Check sheet for the modelled part. Datum: model origin and axes. Units: mm. A direction names the side the tool comes from. Give positions to 0.01 mm unless a question says otherwise; leave off trailing zeros. Order: outer loops, then holes, each group sorted by start corner. A loop starts at its lowest first (then second) coordinate and runs counter-clockwise, first axis right, second up.
```python
from build123d import *

# Parameters (mm, degrees)
SKETCH1_W               = 139.5
SKETCH1_H               = 152.4
BOSS_EXTRUDE1_DEPTH     = 6.35
SKETCH2_W               = 139.5
SKETCH2_H               = 152.4
CUT_EXTRUDE1_DEPTH      = 3.375
SKETCH4_R               = 3.175000001
SKETCH4_R_2             = 3.175
BOSS_EXTRUDE3_DEPTH     = 12.7
SKETCH5_R               = 7.874
CUT_EXTRUDE2_DEPTH      = 16.675
SKETCH6_R               = 2.286
CUT_EXTRUDE3_DEPTH      = 3.975
SKETCH7_R               = 1.27
SKETCH7_W               = 31.75
SKETCH7_H               = 12.7
CUT_EXTRUDE4_DEPTH      = 1
CUT_EXTRUDE4_DEPTH_BACK = 16.675


with BuildPart() as part:
    # Sketch1 → Boss-Extrude1 (new body)
    with BuildSketch(Plane(origin=(0, 0, 0), x_dir=(1, 0, 0), z_dir=(0, 1, 0))):
        with Locations((69.75, 76.2)):
            Rectangle(SKETCH1_W, SKETCH1_H)
    extrude(amount=BOSS_EXTRUDE1_DEPTH)

    # Sketch2 → Cut-Extrude1 (cut)
    with BuildSketch(Plane(origin=(0, 6.35, 0), x_dir=(1, 0, 0), z_dir=(0, 1, 0))):
        with Locations((69.75, 76.2)):
            Rectangle(SKETCH2_W, SKETCH2_H)
    extrude(amount=-CUT_EXTRUDE1_DEPTH, mode=Mode.SUBTRACT)

    # Sketch4 → Boss-Extrude3 (add)
    with BuildSketch(Plane(origin=(0, 0, -152.4), x_dir=(-1, 0, 0), z_dir=(0, 0, -1))):
        with BuildLine():
            Line((-130.61, 9.325), (-130.61, 2.975))
            Line((-130.61, 2.975), (-117.91, 2.975))
            Line((-117.91, 2.975), (-117.91, 9.325))
            ThreePointArc((-117.91, 9.325), (-124.26, 15.675), (-130.61, 9.325))
        make_face()
        with Locations((-124.26, 9.325)):
            Circle(SKETCH4_R, mode=Mode.SUBTRACT)
        with BuildLine():
            Line((-21.59, 9.325), (-21.59, 2.975))
            Line((-21.59, 2.975), (-8.89, 2.975))
            Line((-8.89, 2.975), (-8.89, 9.325))
            ThreePointArc((-8.89, 9.325), (-15.24, 15.675), (-21.59, 9.325))
        make_face()
        with Locations((-15.24, 9.325)):
            Circle(SKETCH4_R_2, mode=Mode.SUBTRACT)
    extrude(amount=-BOSS_EXTRUDE3_DEPTH)

    # Sketch5 → Cut-Extrude2 (cut, through all)
    with BuildSketch(Plane.XZ):
        with Locations((69.75, -114.3)):
            Circle(SKETCH5_R)
    extrude(amount=-CUT_EXTRUDE2_DEPTH, mode=Mode.SUBTRACT)

    # Sketch6 → Cut-Extrude3 (cut, through all)
    with BuildSketch(Plane(origin=(0, 2.975, 0), x_dir=(1, 0, 0), z_dir=(0, 1, 0))):
        with Locations((60.098, 7.62)):
            Circle(SKETCH6_R)
        with Locations((79.402, 7.62)):
            Circle(SKETCH6_R)
    extrude(amount=-CUT_EXTRUDE3_DEPTH, mode=Mode.SUBTRACT)

    # Sketch7 → Cut-Extrude4 (cut, two sides)
    with BuildSketch(Plane.XZ) as cut_extrude4_sk:
        with Locations((46.89, -40.64)):
            Circle(SKETCH7_R)
        with Locations((92.61, -40.64)):
            Circle(SKETCH7_R)
        with Locations((92.61, -58.42)):
            Circle(SKETCH7_R)
        with Locations((46.89, -58.42)):
            Circle(SKETCH7_R)
        with Locations((69.75, -49.53)):
            Rectangle(SKETCH7_W, SKETCH7_H)
    extrude(amount=CUT_EXTRUDE4_DEPTH, mode=Mode.SUBTRACT)
    extrude(cut_extrude4_sk.sketch, amount=-CUT_EXTRUDE4_DEPTH_BACK, mode=Mode.SUBTRACT)


solid = part.part
```
(1) Release check for a two-part mould opening along Z. For faces 1 (the face through (77.26, 1.47, -111.93)), 2 (the face through (69, 2, -152.4)), 3 (the face through (124, 5, -139.7)), 4 (the face through (124.12, 15.673, -146.139)) record: released by +Z, released by -Z, zero draft, split by the parting line, or undercut.
(2) Sectioned sample at A-A (z = -114.3). Enter the section's corners in (x, y) (3 decimals).
(3) Tool access check on faces 5 (the face through (117.91, 6, -146)), 6 (the face through (8.89, 6, -146)), 7 (the face through (130.61, 6, -146)). Record the directions out of +Z, -Z, +X, -X, +Y, -Y that give a thin tool (end or side, any length) a straight path to the whole face; none if there is none.
(4) Go/stop test with flat-tipped pins: P1, Ø1.5, axis at y = 1, z = -51, coming from the -X side; P2, Ø1.9, axis at y = 6.5, z = -143.5, coming from the -X side; P3, Ø3.5, axis at x = 92.61, z = -58.42, coming from the +Y side (3 decimals); P4, Ø5, axis at y = 6, z = -146, coming from the +X side. Record where each tip stops, or that it passes through.
(5) Thickness scan on L1, parallel to X at y = 1.25, z = -7.62; L2, parallel to Z at x = 46.89, y = 1.2; L3, parallel to X at y = 0.5, z = -113.5. Record the ranges inside material, lowest first.
(6) Sectioned sample at B-B (x = 69.75). Enter the section's corners in (y, z) (3 decimals).
(7) Sectioned sample at D-D (x = 124.26). Enter the section's corners in (y, z) (3 decimals).
(8) Sectioned sample at C-C (z = -7.62). Enter the section's corners in (x, y) (3 decimals).
Values follow:
1. face 1: undercut
1. face 2: released by -Z
1. face 3: released by +Z
1. face 4: zero draft
2. outline: (0, 0) - (61.876, 0) - (61.876, 2.975) - (0, 2.975) - close; (77.624, 0) - (139.5, 0) - (139.5, 2.975) - (77.624, 2.975) - close
3. face 5: +Z, -Z, +Y
3. face 6: +Z, -Z, -X, +Y
3. face 7: +Z, -Z, +X, +Y
4. P1: stops at x = 0
4. P2: stops at x = 8.89
4. P3: stops at y = 2.975
4. P4: stops at x = 130.61
5. L1: x = 0 to 57.81, 62.38 to 77.12, 81.69 to 139.5
5. L2: z = -152.4 to -59.69, -57.15 to -41.91, -39.37 to 0
5. L3: x = 0 to 61.92, 77.58 to 139.5
6. outline: (0, -152.4) - (2.975, -152.4) - (2.975, -122.174) - (0, -122.174) - close; (0, -106.426) - (2.975, -106.426) - (2.975, -55.88) - (0, -55.88) - close; (0, -43.18) - (2.975, -43.18) - (2.975, 0) - (0, 0) - close
7. outline: (0, -152.4) - (6.15, -152.4) - (6.15, -139.7) - (2.975, -139.7) - (2.975, 0) - (0, 0) - close; (12.5, -152.4) - (15.675, -152.4) - (15.675, -139.7) - (12.5, -139.7) - close
8. outline: (0, 0) - (57.812, 0) - (57.812, 2.975) - (0, 2.975) - close; (62.384, 0) - (77.116, 0) - (77.116, 2.975) - (62.384, 2.975) - close; (81.688, 0) - (139.5, 0) - (139.5, 2.975) - (81.688, 2.975) - close
